Source: CAD feature listing. Evaluate the final solid. Frame: model axes, mm. A direction names the side the tool comes from. Round coordinates to 2 decimals unless told otherwise and drop trailing zeros. Order: outer loops, then holes, each group sorted by start corner. A loop starts at its lowest first (then second) coordinate and runs counter-clockwise, first axis right, second up. Notation, with made-up numbers: M -10,72.5 L 46,72.5 A11 ccw 46,92.5 Z; hole C 8,37.5 d6. An arc over 180 degrees is marked long. Use CSV: the item, a comma, the result in double quotes. Start each with the question number.
```python
from build123d import *

# Parameters (mm, degrees)
BOSS_EXTRUDE1_DEPTH          = 457.2
BOSS_EXTRUDE1_DEPTH_BACK     = 457.2
F_3_8_0_375_DIAMETER_HOLE1_D = 9.525
F_3_8_0_375_DIAMETER_HOLE2_D = 9.525
SKETCH10_W                   = 777.465907107
SKETCH10_H                   = 78.912238835
CUT_EXTRUDE1_DEPTH           = 33.02


with BuildPart() as part:
    # Sketch4 → Boss-Extrude1 (new, two sides: drawn at the far end of the back side and taken through both)
    with BuildSketch(Plane.XY.offset(-BOSS_EXTRUDE1_DEPTH_BACK)):
        with BuildLine():
            Line((7.9375, -7.14375), (7.9375, 7.14375))
            ThreePointArc((7.9375, 7.14375), (7.705016008, 7.705016008), (7.14375, 7.9375))
            Line((7.14375, 7.9375), (-7.14375, 7.9375))
            ThreePointArc((-7.14375, 7.9375), (-7.705016008, 7.705016008), (-7.9375, 7.14375))
            Line((-7.9375, 7.14375), (-7.9375, -7.14375))
            ThreePointArc((-7.9375, -7.14375), (-7.705016008, -7.705016008), (-7.14375, -7.9375))
            Line((-7.14375, -7.9375), (7.14375, -7.9375))
            ThreePointArc((7.14375, -7.9375), (7.705016008, -7.705016008), (7.9375, -7.14375))
        make_face()
        with BuildLine():
            Line((6.2865, 5.65785), (6.2865, -5.65785))
            ThreePointArc((6.2865, -5.65785), (6.102372678, -6.102372678), (5.65785, -6.2865))
            Line((5.65785, -6.2865), (-5.65785, -6.2865))
            ThreePointArc((-5.65785, -6.2865), (-6.102372678, -6.102372678), (-6.2865, -5.65785))
            Line((-6.2865, -5.65785), (-6.2865, 5.65785))
            ThreePointArc((-6.2865, 5.65785), (-6.102372678, 6.102372678), (-5.65785, 6.2865))
            Line((-5.65785, 6.2865), (5.65785, 6.2865))
            ThreePointArc((5.65785, 6.2865), (6.102372678, 6.102372678), (6.2865, 5.65785))
        make_face(mode=Mode.SUBTRACT)
    extrude(amount=BOSS_EXTRUDE1_DEPTH + BOSS_EXTRUDE1_DEPTH_BACK)

    # 3/8 (0.375) Diameter Hole1 (through all)
    with Locations(Plane(origin=(0, -7.9375, 0), x_dir=(-1, 0, 0), z_dir=(0, -1, 0))):
        with Locations((0, 415.13125)):
            Hole(F_3_8_0_375_DIAMETER_HOLE1_D / 2)

    # 3/8 (0.375) Diameter Hole2 (through all)
    with Locations(Plane(origin=(0, 7.9375, 0), x_dir=(1, 0, 0), z_dir=(0, 1, 0))):
        with Locations((0, 345.28125)):
            Hole(F_3_8_0_375_DIAMETER_HOLE2_D / 2)

    # Sketch10 → Cut-Extrude1 (cut)
    with BuildSketch(Plane.ZY.offset(7.9375)):
        with Locations((219.099444852, 1.446775725)):
            Rectangle(SKETCH10_W, SKETCH10_H)
    extrude(amount=-CUT_EXTRUDE1_DEPTH, mode=Mode.SUBTRACT)


solid = part.part
```
(1) Reachability of faces 1 (the face through (7.938, 0, -315)), 2 (the face through (0, -6.286, -315)) from +Z, -Z, +X, -X, +Y, -Y: full face, straight path, thin tool, end or side. Return the list, or none.
(2) Section C-C on z = -380. Return loops of the section in (x, y), plus the area to 3 significant figures.
(3) Draft query along Z for faces 3 (the face through (-1.03, -7.1, -410.48)), 4 (the face through (-6.286, 0, -315)), 5 (the face through (0, -7, -169.634)). Return one class per face: pulls with the +Z half, pulls with the -Z half, needs draft (parallel to the pull), parting line crosses it, or undercut.
(4) Section B-B on x = 0. Return loops of the section in (y, z), plus the area to 3 significant figures.
(5) Contact query for a flat-ended pin moving along its axis: P1, Ø7.5, axis at x = 0, z = -415.13, coming from the +Y side. Output: stop coordinate, or through.
(6) Line query: line 1 along Z through (x, y) = (0, 7.65); line 2 along Y through (x, z) = (-4, -202.5); line 3 along X through (y, z) = (-5.75, -352). Output: solid intervals per line, ascending.
(7) Section A-A on y = 1. Return loops of the section in (x, z).
Results below:
1,face 1,"+Z, -Z, +X, +Y, -Y"
1,face 2,"+Z, -Z"
2,outline,"M -7.94,-7.14 A0.79 ccw -7.14,-7.94 L 7.14,-7.94 A0.79 ccw 7.94,-7.14 L 7.94,7.14 A0.79 ccw 7.14,7.94 L -7.14,7.94 A0.79 ccw -7.94,7.14 Z; hole M -6.29,-5.66 A0.63 ccw -5.66,-6.29 L 5.66,-6.29 A0.63 ccw 6.29,-5.66 L 6.29,5.66 A0.63 ccw 5.66,6.29 L -5.66,6.29 A0.63 ccw -6.29,5.66 Z"
2,area,"93.7 mm2"
3,face 3,"undercut"
3,face 4,"needs draft"
3,face 5,"pulls with the +Z half"
4,outline,"M -7.94,-457.2 L -6.29,-457.2 L -6.29,-419.89 L -7.94,-419.89 Z; M -7.94,-410.37 L -6.29,-410.37 L -6.29,-350.04 L -7.94,-350.04 Z; M -7.94,-340.52 L -6.29,-340.52 L -6.29,-169.63 L -7.94,-169.63 Z; M 6.29,-457.2 L 7.94,-457.2 L 7.94,-419.89 L 6.29,-419.89 Z; M 6.29,-410.37 L 7.94,-410.37 L 7.94,-350.04 L 6.29,-350.04 Z; M 6.29,-340.52 L 7.94,-340.52 L 7.94,-169.63 L 6.29,-169.63 Z"
4,area,"887 mm2"
5,P1,"passes through"
6,line 1,"z = -457.2 to -419.89, -410.37 to -350.04, -340.52 to -169.63"
6,line 2,"y = -7.94 to -6.29, 6.29 to 7.94"
6,line 3,"x = -7.94 to -6.28, 6.28 to 7.94"
7,outline,"M -7.94,-457.2 L -6.29,-457.2 L -6.29,-169.63 L -7.94,-169.63 Z; M 6.29,-457.2 L 7.94,-457.2 L 7.94,-169.63 L 6.29,-169.63 Z"
